Autodesk Inventor part; units mm, degrees
ref_plane "YZ Plane" through (0, 0, 0) normal (1, 0, 0) x (0, 1, 0)
ref_plane "XZ Plane" through (0, 0, 0) normal (0, 1, 0) x (-1, 0, 0)
ref_plane "XY Plane" through (0, 0, 0) normal (0, 0, 1) x (1, 0, 0)
sketch "Sketch1" plane through (0, 0, 0) normal (0, 1, 0) x (-1, 0, 0)
  line L0 (0, 0) -> (18.15, 0)
  line L1 (18.15, 0) -> (18.15, -13.15)
  line L2 (18.15, -13.15) -> (0, -13.15)
  line L3 (0, -13.15) -> (0, 0)
  dimension "d0" = 18.15
  dimension "d1" = 13.15
extrude "Extrusion1" add sketch "Sketch1" along normal blind 11.5
sketch "Sketch2" plane through (0, 0, 0) normal (0, -1, 0) x (1, 0, 0)
  circle A0 centre (-8.15, -1.475) radius 1.6
  line L0 (0, 0) -> (0, -13.15)
  line L1 (-18.15, -13.15) -> (-18.15, 0)
  line L2 (0, 0) -> (0, -13.15)
  line L3 (0, -6.575) -> (-18.15, -6.575) construction
  circle A1 centre (-8.15, -11.675) radius 1.6
  dimension "d5" = 10
  dimension "d6" = 3.2
  dimension "d7" = 5.1
extrude "Extrusion2" add sketch "Sketch2" along normal blind 3.2
sketch "Sketch3" plane through (0, 0, 0) normal (1, 0, 0) x (0, 0, -1)
  line L0 (0, 0) -> (13.15, 0)
  line L1 (6.575, 0) -> (6.575, 11.5) construction
  line L2 (13.15, 11.5) -> (0, 11.5)
  line L3 (3.075, 0) -> (3.075, 3)
  line L4 (3.075, 3) -> (1.075, 3)
  line L5 (1.075, 3) -> (1.075, 10)
  line L6 (1.075, 10) -> (3.075, 10)
  line L7 (3.075, 10) -> (3.075, 10.2)
  line L8 (3.075, 10.2) -> (6.575, 10.2)
  line L9 (3.075, 0) -> (6.575, 0)
  line L10 (10.075, 0) -> (10.075, 3)
  line L11 (10.075, 3) -> (12.075, 3)
  line L12 (12.075, 3) -> (12.075, 10)
  line L13 (12.075, 10) -> (10.075, 10)
  line L14 (10.075, 10) -> (10.075, 10.2)
  line L15 (10.075, 10.2) -> (6.575, 10.2)
  line L16 (10.075, 0) -> (6.575, 0)
  dimension "d10" = 3.5
  dimension "d11" = 3
  dimension "d12" = 7
  dimension "d13" = 2
  dimension "d15" = 1.3
extrude "Extrusion3" cut sketch "Sketch3" against normal blind 13
fillet "Fillet1" radius 0.5 8 edges at (0, 5.75, -13.15) (-9.075, 11.5, -13.15) (0, 11.5, -6.575) (0, 5.75, 0) (-9.075, 11.5, 0) (-18.15, 5.75, 0) (-18.15, 11.5, -6.575) (-18.15, 5.75, -13.15)
properties part number "RJ12 Connector"
Source: CAD feature listing. Evaluate the final solid. Frame: model axes, mm. A direction names the side the tool comes from. Give positions to 0.01 mm unless a question says otherwise; leave off trailing zeros. Write each loop counter-clockwise with the first axis right and the second up, starting at its lowest first coordinate (ties: lowest second). Pieces come first, ordered by that corner, then holes. Notation, with made-up numbers: (84, 80.25) - (112, 80.25) arc R19 cw to (112, 97.25) - close; hole circle Ø9 at (0.25, -26.75). An arc over 180 degrees is marked (long way). One line per item, written item: value. Start each with the question number.
Q1. Material intervals for probe 1 along Y at (x, z) = (-1, -10.25); probe 2 along Z at (x, y) = (-3.25, 2.75) (3 decimals); probe 3 along Z at (x, y) = (-10.5, 3.5) (3 decimals), sorted ascending. Write a range as from..to.
Q2. Section query B-B, the plane x = -2. Return the cut outline in (y, z) (3 decimals).
Q3. Section query C-C, the plane z = -6.75. Return the cut outline in (x, y), then the cut area to 3 significant figures.
Q4. Set-up query: faces 1 (the face through (-6, 6, -12.075)), 2 (the face through (-8, -3.2, -12)), 3 (the face through (0, 2.6, -10.7)), 4 (the face through (-9.42, -1.58, -0.5)), 5 (the face through (-6, 10.2, -7)). Return all of +Z, -Z, +X, -X, +Y, -Y with unobstructed straight access to the full face (end or side cutting, diameter ignored); none if empty.
Q5. Section query A-A, the plane y = 10.75. Return the cut outline in (x, z).
Q6. First-contact query: pin 1 Ø0.9 at (x, z) = (-3.5, -2) entering from -Y; pin 2 Ø2.5 at (x, y) = (-5, 1) entering from -Z; pin 3 Ø7.5 at (x, z) = (-6.5, -8) entering from -Y; pin 4 Ø3.5 at (x, y) = (-9, 3) entering from +Z. Flat tips, straight axial feed; report the tip coordinate or a pass-through.
Q7. Draft query along Y for faces 6 (the face through (-8, -3.2, -1)), 7 (the face through (-9.329, -1.578, -12.756)), 8 (the face through (-6, 10, -11)). Return one class per face: +Y half, -Y half, draft (parallel to the pull), parting line (faces both ways), or undercut.
Q8. Section query D-D, the plane y = 8. Return the cut outline in (x, z) (3 decimals), then the cut area to 3 significant figures.
Answer:
1. probe 1: y = 0..3, 10..11.5
1. probe 2: z = -13.15..-10.075, -3.075..0
1. probe 3: z = -13.15..-12.075, -1.075..0
2. outline: (0, -13.15) - (11, -13.15) arc R0.5 ccw to (11.5, -12.65) - (11.5, -0.5) arc R0.5 ccw to (11, 0) - (0, 0) - (0, -3.075) - (3, -3.075) - (3, -1.075) - (10, -1.075) - (10, -3.075) - (10.2, -3.075) - (10.2, -10.075) - (10, -10.075) - (10, -12.075) - (3, -12.075) - (3, -10.075) - (0, -10.075) - close
3. outline: (-18.15, 0) - (-13, 0) - (-13, 10.2) - (0, 10.2) - (0, 11) arc R0.5 ccw to (-0.5, 11.5) - (-17.65, 11.5) arc R0.5 ccw to (-18.15, 11) - close
3. area: 76.0 mm2
4. face 1: +X
4. face 2: +Z, -Z, +X, -X, -Y
4. face 3: +Z, -Z, +X, +Y, -Y
4. face 4: -Y
4. face 5: +X, -Y
5. outline: (-18.15, -12.65) arc R0.5 ccw to (-17.65, -13.15) - (-0.5, -13.15) arc R0.5 ccw to (0, -12.65) - (0, -0.5) arc R0.5 ccw to (-0.5, 0) - (-17.65, 0) arc R0.5 ccw to (-18.15, -0.5) - close
6. pin 1: stops at y = 0
6. pin 2: stops at z = -13.15
6. pin 3: stops at y = -3.2
6. pin 4: stops at z = 0
7. face 6: -Y half
7. face 7: draft
7. face 8: undercut
8. outline: (-18.15, -12.65) arc R0.5 ccw to (-17.65, -13.15) - (-0.5, -13.15) arc R0.5 ccw to (0, -12.65) - (0, -12.075) - (-13, -12.075) - (-13, -1.075) - (0, -1.075) - (0, -0.5) arc R0.5 ccw to (-0.5, 0) - (-17.65, 0) arc R0.5 ccw to (-18.15, -0.5) - close
8. area: 95.5 mm2
